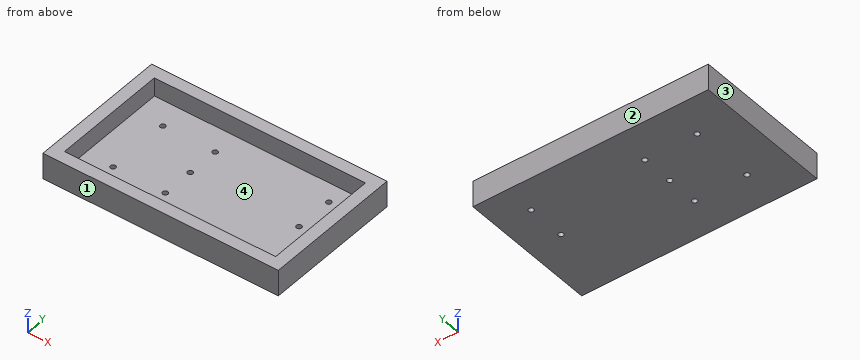
```python
from build123d import *

# Parameters (mm, degrees)
SKETCH1_W           = 135
SKETCH1_H           = 80
BOSS_EXTRUDE1_DEPTH = 40
SKETCH2_R           = 1.5
CUT_EXTRUDE1_DEPTH  = 10
SKETCH4_W           = 135
SKETCH4_H           = 25
CUT_EXTRUDE2_DEPTH  = 100


with BuildPart() as part:
    # Sketch1 → Boss-Extrude1 (new body)
    with BuildSketch(Plane.XY):
        with Locations((67.5, 40)):
            Rectangle(SKETCH1_W, SKETCH1_H)
    extrude(amount=-BOSS_EXTRUDE1_DEPTH)

    # Sketch2 → Cut-Extrude1 (cut)
    with BuildSketch(Plane(origin=(0, 0, -40), x_dir=(-1, 0, 0), z_dir=(0, 0, -1))):
        with Locations((-53.3, 40)):
            Circle(SKETCH2_R)
        with Locations((-53.3, 58.35)):
            Circle(SKETCH2_R)
        with Locations((-53.3, 21.65)):
            Circle(SKETCH2_R)
        with Locations((-23.3, 58.35)):
            Circle(SKETCH2_R)
        with Locations((-23.3, 21.65)):
            Circle(SKETCH2_R)
        with Locations((-115.7, 40)):
            Circle(SKETCH2_R)
        with Locations((-115.7, 62)):
            Circle(SKETCH2_R)
    extrude(amount=-CUT_EXTRUDE1_DEPTH, mode=Mode.SUBTRACT)

    # Cavity1: read off the stored shape, not the designer's step
    # Cavity1: loft between two sections, ruled curve by curve
    cavity1_from = [
        Edge.make_line((128.706, 6.25125, 0), (128.706, 73.74875, 0)),
        Edge.make_line((6.294, 6.25125, 0), (128.706, 6.25125, 0)),
        Edge.make_line((6.294, 73.74875, 0), (6.294, 6.25125, 0)),
        Edge.make_line((128.706, 73.74875, 0), (6.294, 73.74875, 0)),
    ]
    cavity1_to = [
        Edge.make_line((127.780327673, 7.181504864, -35.35), (127.780327673, 72.818495136, -35.35)),
        Edge.make_line((7.219672327, 7.181504864, -35.35), (127.780327673, 7.181504864, -35.35)),
        Edge.make_line((7.219672327, 72.818495136, -35.35), (7.219672327, 7.181504864, -35.35)),
        Edge.make_line((127.780327673, 72.818495136, -35.35), (7.219672327, 72.818495136, -35.35)),
    ]
    cavity1 = Solid(Shell([*[Face.make_surface_from_curves(cavity1_from[k], cavity1_to[k]) for k in range(4)], Face(Wire(cavity1_from)), Face(Wire(cavity1_to))]))
    add(cavity1, mode=Mode.SUBTRACT)

    # Sketch4 → Cut-Extrude2 (cut)
    with BuildSketch(Plane(origin=(0, 80, 0), x_dir=(1, 0, 0), z_dir=(0, 1, 0))):
        with Locations((67.5, 12.5)):
            Rectangle(SKETCH4_W, SKETCH4_H)
    extrude(amount=-CUT_EXTRUDE2_DEPTH, mode=Mode.SUBTRACT)


solid = part.part
```
The listing builds one solid part. Answer for the finished solid, in the listing's coordinates (mm). Face numbers are marked on the shaded views. Give positions to 0.01 mm unless a question says otherwise; leave off trailing zeros. Write item = value, one per line. Start each with the question number.
1) Straight lines are drawn through the part: line 1 along Y through (x, z) = (23.3, -38.7); line 2 along Y through (x, z) = (53.3, -36.8); line 3 along Y through (x, z) = (115.7, -38). For each, find the intervals that lie inside material, in ascending order.
2) This flat-tipped pin is pushed along its axis until it touches: pin 1 (1.5 mm diameter, centred on x = 81, y = 62, fed in from +Z). Where does it stop, or does it pass through?
3) The part is cut by section A-A, the plane x = 53.3. Count the separate pieces of the cut face and the enclosed holes in it, and give its area (3 significant figures).
4) Determine the mould class of the marked faces 1, 2, 3 and 4 for opening direction Y: +Y half, -Y half, draft (parallel to the pull), parting line (faces both ways), or undercut.
Solutions:
q1.line_1 = 0 to 20.15, 23.15 to 56.85, 59.85 to 80
q1.line_2 = 0 to 20.15, 23.15 to 38.5, 41.5 to 56.85, 59.85 to 80
q1.line_3 = 0 to 38.5, 41.5 to 60.5, 63.5 to 80
q2.pin_1 = -35.35
q3.separate_pieces = 4
q3.enclosed_holes = 0
q3.area = 476 mm²
q4.face_1 = -Y half
q4.face_2 = +Y half
q4.face_3 = draft
q4.face_4 = undercut
